CAD build for the part. Positions are in the model's coordinates, mm. A direction names the side the tool comes from. Give positions to 0.01 mm unless a question says otherwise; leave off trailing zeros. Order: outer loops, then holes, each group sorted by start corner. A loop starts at its lowest first (then second) coordinate and runs counter-clockwise, first axis right, second up.
```python
from build123d import *

# Parameters (mm, degrees)
BOSS_EXTRUDE1_DEPTH = 80
BOSS_EXTRUDE2_DEPTH = 10


with BuildPart() as part:
    # Sketch1 → Boss-Extrude1 (new, symmetric)
    with BuildSketch(Plane(origin=(0, 0, 0), x_dir=(1, 0, 0), z_dir=(0, 1, 0))):
        Polygon((0, -40.082250377), (70.710678119, -110.792928496), (63.639610307, -117.863996308), (0, -54.224386001), (-63.639610307, -117.863996308), (-70.710678119, -110.792928496), align=None)
    extrude(amount=BOSS_EXTRUDE1_DEPTH, both=True)

    # Sketch2 → Boss-Extrude2 (add)
    with BuildSketch(Plane.XZ.offset(80)):
        Polygon((-63.639610307, 117.863996308), (0, 54.224386001), (63.639610307, 117.863996308), (25, 156.503606614), (-25, 156.503606614), align=None)
    extrude(amount=-BOSS_EXTRUDE2_DEPTH)


solid = part.part
```
Item 1: Slice it at C-C (x = 10). Give the cut face in (y, z), and give its area (3 significant figures).
Item 2: Tool access for faces 1 (the face through (11, 80, 64)), 2 (the face through (-1, -70, 117)): list every direction of +Z, -Z, +X, -X, +Y, -Y with a clear straight run to the whole face (end or side of a thin tool).
Item 3: Two-plate mould, pull along X, no slides. Class faces 3 (the face through (32.265, 6.05, 86.49)), 4 (the face through (-1, -80, 112)), 5 (the face through (-35.85, 1.12, 75.93)): released by +X, released by -X, zero draft, split by the parting line, or undercut.
Item 4: Slice it at B-B (y = -43). Give the cut face in (x, z).
Item 5: Slice it at D-D (z = 94.5). Give the cut face in (x, y).
Item 6: Drop flat-ended pins along their axis: pin 1 Ø4 at (x, y) = (-34, 6) entering from +Z; pin 2 Ø4 at (y, z) = (31.5, 118.5) entering from -X; pin 3 Ø4 at (x, y) = (33, 50.5) entering from -Z. Give the stop position or say it passes through.
Item 7: Slice it at A-A (z = 80). Give the cut face in (x, y), and give its area (3 significant figures).
Item 8: Wall check: L1, parallel to Y at x = 26.5, z = 113.5; L2, parallel to X at y = 50, z = 91.5; L3, parallel to X at y = -34.5, z = 79. Give the ranges that are in metal, low to high.
A:
1. outline: (-80, 50.08) - (80, 50.08) - (80, 64.22) - (-70, 64.22) - (-70, 156.5) - (-80, 156.5) - close
1. area: 3,190 mm2
2. face 1: +Z, -Z, +X, -X, +Y
2. face 2: +Z, +Y
3. face 3: undercut
3. face 4: zero draft
3. face 5: released by -X
4. outline: (-70.71, 110.79) - (0, 40.08) - (70.71, 110.79) - (63.64, 117.86) - (0, 54.22) - (-63.64, 117.86) - close
5. outline: (-54.42, -80) - (54.42, -80) - (54.42, 80) - (40.28, 80) - (40.28, -70) - (-40.28, -70) - (-40.28, 80) - (-54.42, 80) - close
6. pin 1: stops at z = 90.22
6. pin 2: stops at x = -65
6. pin 3: stops at z = 71.08
7. outline: (-39.92, -80) - (39.92, -80) - (39.92, 80) - (25.78, 80) - (25.78, -70) - (-25.78, -70) - (-25.78, 80) - (-39.92, 80) - close
7. area: 5,040 mm2
8. L1: y = -80 to -70
8. L2: x = -51.42 to -37.28, 37.28 to 51.42
8. L3: x = -38.92 to -24.78, 24.78 to 38.92
